```python
from build123d import *

# Parameters (mm, degrees)
PAD_DEPTH        = 19.05
HOLE_D           = 4.5
HOLE_DEPTH       = 14.986
HOLE_CSINK_D     = 6.985
HOLE_CSINK_ANGLE = 82
HOLE_TIPS_R      = 2.25
SKETCH002_W      = 25.4
SKETCH002_H      = 49.53
POCKET_DEPTH     = 10.16
FILLET_R         = 0.508
CHAMFER_SIZE     = 0.254


with BuildPart() as part:
    # Sketch → Pad (new body)
    with BuildSketch(Plane.XY):
        with BuildLine():
            Line((-62.570064, -20.660064), (-59.395064, -23.835064))
            ThreePointArc((-59.395064, -23.835064), (-58.36502, -24.523318), (-57.15, -24.765))
            Line((-57.15, -24.765), (57.15, -24.765))
            ThreePointArc((57.15, -24.765), (58.36502, -24.523318), (59.395064, -23.835064))
            Line((59.395064, -23.835064), (62.570064, -20.660064))
            ThreePointArc((62.570064, -20.660064), (63.258318, -19.63002), (63.5, -18.415))
            Line((63.5, -18.415), (63.5, 18.415))
            ThreePointArc((63.5, 18.415), (63.258318, 19.63002), (62.570064, 20.660064))
            Line((62.570064, 20.660064), (59.395064, 23.835064))
            ThreePointArc((59.395064, 23.835064), (58.36502, 24.523318), (57.15, 24.765))
            Line((57.15, 24.765), (-57.15, 24.765))
            ThreePointArc((-57.15, 24.765), (-58.36502, 24.523318), (-59.395064, 23.835064))
            Line((-59.395064, 23.835064), (-62.570064, 20.660064))
            ThreePointArc((-62.570064, 20.660064), (-63.258318, 19.63002), (-63.5, 18.415))
            Line((-63.5, 18.415), (-63.5, -18.415))
            ThreePointArc((-63.5, -18.415), (-63.258318, -19.63002), (-62.570064, -20.660064))
        make_face()
    extrude(amount=PAD_DEPTH)

    # Hole
    with Locations(Plane.XY.offset(19.05)):
        with Locations((-9.525, 15.875), (9.525, 15.875), (12.7, 0), (-12.7, 0), (-9.525, -15.875), (9.525, -15.875)):
            CounterSinkHole(HOLE_D / 2, HOLE_CSINK_D / 2, depth=HOLE_DEPTH, counter_sink_angle=HOLE_CSINK_ANGLE)

    # Hole tips → Hole tip 1 section 0
    with BuildSketch(Plane.XY.offset(4.064), mode=Mode.PRIVATE) as hole_tip_1_s0:
        with Locations((-9.525, 15.875)):
            Circle(HOLE_TIPS_R)
    loft([hole_tip_1_s0.sketch, Vertex(-9.525, 15.875, 2.712064)], mode=Mode.SUBTRACT)

    # Hole tips → Hole tip 2 section 0
    with BuildSketch(Plane.XY.offset(4.064), mode=Mode.PRIVATE) as hole_tip_2_s0:
        with Locations((9.525, 15.875)):
            Circle(HOLE_TIPS_R)
    loft([hole_tip_2_s0.sketch, Vertex(9.525, 15.875, 2.712064)], mode=Mode.SUBTRACT)

    # Hole tips → Hole tip 3 section 0
    with BuildSketch(Plane.XY.offset(4.064), mode=Mode.PRIVATE) as hole_tip_3_s0:
        with Locations((12.7, 0)):
            Circle(HOLE_TIPS_R)
    loft([hole_tip_3_s0.sketch, Vertex(12.7, 0, 2.712064)], mode=Mode.SUBTRACT)

    # Hole tips → Hole tip 4 section 0
    with BuildSketch(Plane.XY.offset(4.064), mode=Mode.PRIVATE) as hole_tip_4_s0:
        with Locations((-12.7, 0)):
            Circle(HOLE_TIPS_R)
    loft([hole_tip_4_s0.sketch, Vertex(-12.7, 0, 2.712064)], mode=Mode.SUBTRACT)

    # Hole tips → Hole tip 5 section 0
    with BuildSketch(Plane.XY.offset(4.064), mode=Mode.PRIVATE) as hole_tip_5_s0:
        with Locations((-9.525, -15.875)):
            Circle(HOLE_TIPS_R)
    loft([hole_tip_5_s0.sketch, Vertex(-9.525, -15.875, 2.712064)], mode=Mode.SUBTRACT)

    # Hole tips → Hole tip 6 section 0
    with BuildSketch(Plane.XY.offset(4.064), mode=Mode.PRIVATE) as hole_tip_6_s0:
        with Locations((9.525, -15.875)):
            Circle(HOLE_TIPS_R)
    loft([hole_tip_6_s0.sketch, Vertex(9.525, -15.875, 2.712064)], mode=Mode.SUBTRACT)

    # Sketch002 (on Face5 of Hole) → Pocket (cut)
    with BuildSketch(Plane.XY.offset(19.05)):
        with Locations((-38.1, 0)):
            Rectangle(SKETCH002_W, SKETCH002_H)
        with Locations((38.1, 0)):
            Rectangle(SKETCH002_W, SKETCH002_H)
    extrude(amount=-POCKET_DEPTH, mode=Mode.SUBTRACT)

    # Fillet
    fillet_edges = [part.edges().sort_by_distance(p)[0] for p in [
        (-50.8, -24.765, 13.97),
        (-50.8, 24.765, 13.97),
        (-25.4, -24.765, 13.97),
        (25.4, -24.765, 13.97),
        (50.8, -24.765, 13.97),
        (50.8, 24.765, 13.97),
        (25.4, 24.765, 13.97),
        (-25.4, 24.765, 13.97),
    ]]
    fillet(fillet_edges, radius=FILLET_R)

    # Chamfer
    chamfer_edges = [part.edges().sort_by_distance(p)[0] for p in [
        (54.229, 24.765, 19.05),
        (0, 24.765, 19.05),
        (-54.229, 24.765, 19.05),
    ]]
    chamfer(chamfer_edges, length=CHAMFER_SIZE)


solid = part.part
```
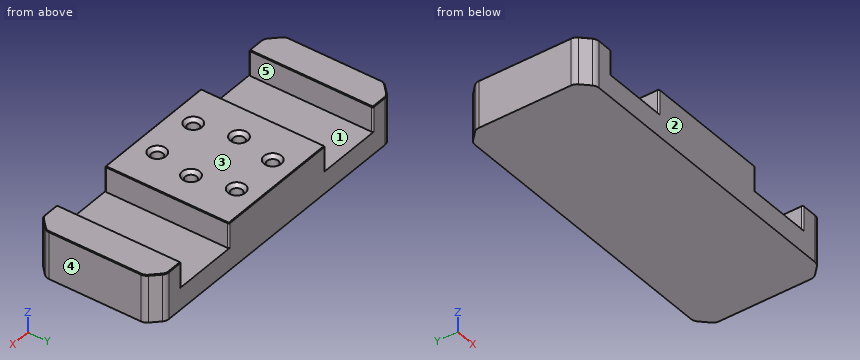
CAD build for the part. Positions are in the model's coordinates, mm. Face numbers are marked on the shaded views. A direction names the side the tool comes from. Give positions to 0.01 mm unless a question says otherwise; leave off trailing zeros. Loops run counter-clockwise (first coordinate to the right, second up) from the corner with the lowest first, then second, coordinate; pieces in that order, holes last. Notation, with made-up numbers: (-11, -26.5) - (11, -26.5) arc R14 cw to (11, -0.5) - close; hole circle Ø4 at (52.5, 26.5). An arc over 180 degrees is marked (long way). Put each result on its own line as item: value.
Q1. Slice it at C-C (z = 11). Give the number of separate pieces and of enclosed holes in the cut face, plus the area to 3 significant figures.
Filled in:
separate pieces: 3
enclosed holes: 6
area: 3,630 mm²
Q2. Slice it at A-A (z = 5.25). Give the cut face in (x, y) (3 decimals), plus the area to 3 significant figures.
Filled in:
outline: (-63.5, -18.415) arc R3.175 ccw to (-62.57, -20.66) - (-59.395, -23.835) arc R3.175 ccw to (-57.15, -24.765) - (57.15, -24.765) arc R3.175 ccw to (59.395, -23.835) - (62.57, -20.66) arc R3.175 ccw to (63.5, -18.415) - (63.5, 18.415) arc R3.175 ccw to (62.57, 20.66) - (59.395, 23.835) arc R3.175 ccw to (57.15, 24.765) - (-57.15, 24.765) arc R3.175 ccw to (-59.395, 23.835) - (-62.57, 20.66) arc R3.175 ccw to (-63.5, 18.415) - close; hole circle Ø4.5 at (-12.7, 0); hole circle Ø4.5 at (-9.525, -15.875); hole circle Ø4.5 at (-9.525, 15.875); hole circle Ø4.5 at (9.525, -15.875); hole circle Ø4.5 at (9.525, 15.875); hole circle Ø4.5 at (12.7, 0)
area: 6,140 mm²
Q3. Mould opens along X. For the marked faces 3, 4 and 5 say: pulls with the +X half, pulls with the -X half, needs draft (parallel to the pull), parting line crosses it, or undercut.
Filled in:
face 3: needs draft
face 4: pulls with the +X half
face 5: undercut
Q4. Flat gauge pins, fed straight in: pin 1 (1 mm diameter, centred on x = -31, y = 14.5, fed in from +Z); pin 2 (6 mm diameter, centred on x = -9.525, y = 15.875, fed in from +Z); pin 3 (5 mm diameter, centred on x = -12.7, y = 0, fed in from +Z). Where does each tip first touch, or does it go through?
Filled in:
pin 1: stops at z = 8.89
pin 2: stops at z = 18.48
pin 3: stops at z = 17.91
Q5. Slice it at B-B (x = 47). Give the cut face in (y, z) (3 decimals), plus the area to 3 significant figures.
Filled in:
outline: (-24.765, 0) - (24.765, 0) - (24.765, 8.89) - (-24.765, 8.89) - close
area: 440 mm²
Q6. Probe line 1 along X through (y, z) = (12, 11.75); line 2 along X through (y, z) = (0, 14); line 3 along X through (y, z) = (14, 8). List the from-to ranges inside material, lowest first.
Filled in:
line 1: x = -63.5 to -50.8, -25.4 to 25.4, 50.8 to 63.5
line 2: x = -63.5 to -50.8, -25.4 to -14.95, -10.45 to 10.45, 14.95 to 25.4, 50.8 to 63.5
line 3: x = -63.5 to -10.77, -8.28 to 8.28, 10.77 to 63.5
Q7. Tool access for the marked faces 1 and 2: list every direction of +Z, -Z, +X, -X, +Y, -Y with a clear straight run to the whole face (end or side of a thin tool).
Filled in:
face 1: +Z, +Y, -Y
face 2: +Z, -Z, +X, -X, -Y
